```python
from build123d import *

# Parameters (mm, degrees)
BOSS_EXTRUDE1_DEPTH              = 3.175
F_10_0_1935_DIAMETER_HOLE1_D     = 4.9149
F_10_0_1935_DIAMETER_HOLE1_DEPTH = 9.699415072
F_10_0_1935_DIAMETER_HOLE1_TIP   = 1.476584928
FILLET1_R                        = 3.175


with BuildPart() as part:
    # Sketch1 → Boss-Extrude1 (new body)
    with BuildSketch(Plane(origin=(0, 0, 0), x_dir=(0, 0, -1), z_dir=(1, 0, 0))):
        with BuildLine():
            Line((-25.4, 11.1125), (22.225, 11.1125))
            Line((22.225, 11.1125), (22.225, -17.010023672))
            ThreePointArc((22.225, -17.010023672), (21.479421476, -17.696337769), (20.681497174, -18.321022636))
            ThreePointArc((20.681497174, -18.321022636), (20.108002708, -18.71085711), (19.51408533, -19.068808178))
            ThreePointArc((19.51408533, -19.068808178), (16.492659011, -20.297805158), (13.257849362, -20.716681165))
            Line((13.257849362, -20.716681165), (-25.4, -20.716681165))
            Line((-25.4, -20.716681165), (-25.4, 11.1125))
        make_face()
    extrude(amount=BOSS_EXTRUDE1_DEPTH)

    # #10 (0.1935) Diameter Hole1
    with Locations(Plane.ZY):
        with Locations((19.05, 4.7625), (19.05, -15.5575), (0, -5.3975)):
            Hole(F_10_0_1935_DIAMETER_HOLE1_D / 2, depth=F_10_0_1935_DIAMETER_HOLE1_DEPTH)
            with Locations((0, 0, -(F_10_0_1935_DIAMETER_HOLE1_DEPTH + F_10_0_1935_DIAMETER_HOLE1_TIP / 2))):  # 118° drill point
                Cone(0, F_10_0_1935_DIAMETER_HOLE1_D / 2, F_10_0_1935_DIAMETER_HOLE1_TIP, mode=Mode.SUBTRACT)

    # Fillet1
    fillet1_edges = [part.edges().sort_by_distance(p)[0] for p in [
        (1.5875, 11.1125, 25.4),
        (1.5875, 11.1125, -22.225),
        (1.5875, -20.716681165, 25.4),
    ]]
    fillet(fillet1_edges, radius=FILLET1_R)


solid = part.part
```
Read the model definition and answer for the solid it produces. Units are mm, in the model's axes. Coordinates: 2 decimals unless noted, no trailing zeros. Write each loop counter-clockwise with the first axis right and the second up, starting at its lowest first coordinate (ties: lowest second). Pieces come first, ordered by that corner, then holes. Notation, with made-up numbers: (-4, 74) -> (7, 74) arc R12 cw to (7, 93) -> close; hole circle Ø3 at (57.25, -29.5). An arc over 180 degrees is marked (long way). Write item = value, one per line.
(1) Given pin 1 Ø8 at (y, z) = (0, 20.5) entering from -X; pin 2 Ø3 at (y, z) = (-15.56, 19.05) entering from +X, each flat-ended and moving along its own axis, determine where each tip first touches the part or whether it passes through.
From the geometry:
pin_1 = 0
pin_2 = through
(2) Section C-C on z = 19.05 is taken. Write down the section's boundary in (x, y) (1 decimal), plus the area to 3 significant figures.
From the geometry:
outline = (0, -20.7) -> (3.2, -20.7) -> (3.2, -18) -> (0, -18) -> close; (0, -13.1) -> (3.2, -13.1) -> (3.2, 2.3) -> (0, 2.3) -> close; (0, 7.2) -> (3.2, 7.2) -> (3.2, 11.1) -> (0, 11.1) -> close
area = 69.8 mm2
(3) Section D-D on x = 1.2 is taken. Count the separate pieces of the cut face and the enclosed holes in it, plus the area to 3 significant figures.
From the geometry:
separate_pieces = 1
enclosed_holes = 3
area = 1,440 mm2
(4) Section B-B on y = 5.5 is taken. Write down the section's boundary in (x, z) (3 decimals).
From the geometry:
outline = (0, -22.225) -> (3.175, -22.225) -> (3.175, 16.706) -> (0, 16.706) -> close; (0, 21.394) -> (3.175, 21.394) -> (3.175, 25.4) -> (0, 25.4) -> close
(5) Straight lines are drawn through the part: L1, parallel to Y at x = 2.3, z = 19.05; L2, parallel to Y at x = 1.95, z = 0; L3, parallel to Z at x = 1.25, y = -14 (3 decimals). For each, find the intervals that lie inside material, in ascending order. Write a range as from..to.
From the geometry:
L1 = -20.72..-18.01, -13.1..2.31, 7.22..11.11
L2 = -20.72..-7.85, -2.94..11.11
L3 = -22.225..17.149, 20.951..25.4
(6) Section A-A on z = 0 is taken. Write down the section's boundary in (x, y) (1 decimal).
From the geometry:
outline = (0, -20.7) -> (3.2, -20.7) -> (3.2, -7.9) -> (0, -7.9) -> close; (0, -2.9) -> (3.2, -2.9) -> (3.2, 11.1) -> (0, 11.1) -> close
(7) For a pull along Z with two mould halves and no side action, classify faces 1 (the face through (2, 11.112, 2)), 2 (the face through (2, -4, -22.225)), 3 (the face through (1.61, -14.819, 16.706)) as +Z half, -Z half, draft (parallel to the pull), parting line (faces both ways), or undercut.
From the geometry:
face_1 = draft
face_2 = -Z half
face_3 = undercut
